from build123d import *

# Parameters (mm, degrees)
SKETCH_1_W          = 20
SKETCH_1_H          = 20
EXTRUDE_1_DEPTH     = 100
SKETCH_2_R          = 2.1
CUT_EXTRUDE_1_DEPTH = 100
SKETCH_3_R          = 2.1
CUT_EXTRUDE_2_DEPTH = 103.46950766


with BuildPart() as part:
    # 草图1 → 凸台-拉伸1 (new body)
    with BuildSketch(Plane(origin=(0, 0, 0), x_dir=(0, 0, -1), z_dir=(1, 0, 0))):
        Rectangle(SKETCH_1_W, SKETCH_1_H)
    extrude(amount=EXTRUDE_1_DEPTH)

    # 草图2 → 切除-拉伸1 (cut)
    with BuildSketch(Plane.XY.offset(10)):
        with Locations((10, 0)):
            Circle(SKETCH_2_R)
        with Locations((30, 0)):
            Circle(SKETCH_2_R)
        with Locations((50, 0)):
            Circle(SKETCH_2_R)
        with Locations((70, 0)):
            Circle(SKETCH_2_R)
        with Locations((90, 0)):
            Circle(SKETCH_2_R)
    extrude(amount=-CUT_EXTRUDE_1_DEPTH, mode=Mode.SUBTRACT)

    # 草图3 → 切除-拉伸2 (cut, through all)
    with BuildSketch(Plane(origin=(0, 10, 0), x_dir=(1, 0, 0), z_dir=(0, 1, 0))):
        with Locations(Location((10, 0, 0), (0, 0, 270))):
            Circle(SKETCH_3_R)
        with Locations(Location((30, 0, 0), (0, 0, 270))):
            Circle(SKETCH_3_R)
        with Locations(Location((50, 0, 0), (0, 0, 270))):
            Circle(SKETCH_3_R)
        with Locations(Location((70, 0, 0), (0, 0, 270))):
            Circle(SKETCH_3_R)
        with Locations(Location((90, 0, 0), (0, 0, 270))):
            Circle(SKETCH_3_R)
    extrude(amount=-CUT_EXTRUDE_2_DEPTH, mode=Mode.SUBTRACT)


solid = part.part
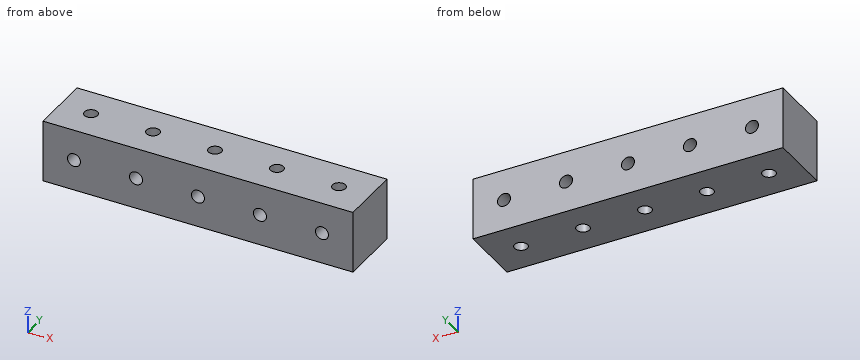
Check sheet for the modelled part. Datum: model origin and axes. Units: mm. Give positions to 0.01 mm unless a question says otherwise; leave off trailing zeros. Loops run counter-clockwise (first coordinate to the right, second up) from the corner with the lowest first, then second, coordinate; pieces in that order, holes last. Notation, with made-up numbers: M 17.5,-14 L 41.5,-14 A34 ccw 41.5,24 Z; hole C 21.5,42 d1. An arc over 180 degrees is marked long. Use a Markdown table: item, result. Add a question column.
Q1. Sectioned sample at B-B, the plane z = -7.75. Record the cut outline in (x, y), then the cut area to 3 significant figures.
Q2. Scan lines: line 1 along X through (y, z) = (8, 0); line 2 along Z through (x, y) = (50, 7.25). Record each from-to range of solid material in increasing order. Write a range as [from, to].
Q3. Sectioned sample at A-A, the plane x = 30. Record the cut outline in (y, z).
Verdict:
| question | item | result |
|---|---|---|
| 1 | outline | M 0,-10 L 100,-10 L 100,10 L 0,10 Z; hole C 10,0 d4.2; hole C 30,0 d4.2; hole C 50,0 d4.2; hole C 70,0 d4.2; hole C 90,0 d4.2 |
| 1 | area | 1,930 mm^2 |
| 2 | line 1 | [0, 7.9], [12.1, 27.9], [32.1, 47.9], [52.1, 67.9], [72.1, 87.9], [92.1, 100] |
| 2 | line 2 | [-10, -2.1], [2.1, 10] |
| 3 | outline | M -10,-10 L -2.1,-10 L -2.1,-2.1 L -10,-2.1 Z; M -10,2.1 L -2.1,2.1 L -2.1,10 L -10,10 Z; M 2.1,-10 L 10,-10 L 10,-2.1 L 2.1,-2.1 Z; M 2.1,2.1 L 10,2.1 L 10,10 L 2.1,10 Z |
